Autodesk Inventor part; units mm, degrees
ref_plane "YZ Plane" through (0, 0, 0) normal (1, 0, 0) x (0, 1, 0)
ref_plane "XZ Plane" through (0, 0, 0) normal (0, 1, 0) x (-1, 0, 0)
ref_plane "XY Plane" through (0, 0, 0) normal (0, 0, 1) x (1, 0, 0)
sketch "Sketch1" plane through (0, 0, 0) normal (1, 0, 0) x (0, 1, 0)
  line L0 (0, 0) -> (39.8649, 0)
  line L1 (39.8649, 0) -> (39.8649, -16.6447)
  line L2 (39.8649, -16.6447) -> (37.3249, -16.6447)
  line L3 (37.3249, -16.6447) -> (37.3249, -5.715)
  line L4 (34.1499, -2.54) -> (0, -2.54)
  line L5 (0, -2.54) -> (0, 0)
  arc A0 (37.3249, -5.715) -> (34.1499, -2.54) centre (34.1499, -5.715) ccw
  dimension "d0" = 2.54
  dimension "d1" = 3.175
extrude "Extrusion1" add sketch "Sketch1" along normal blind 2.54
properties part number "allen key"
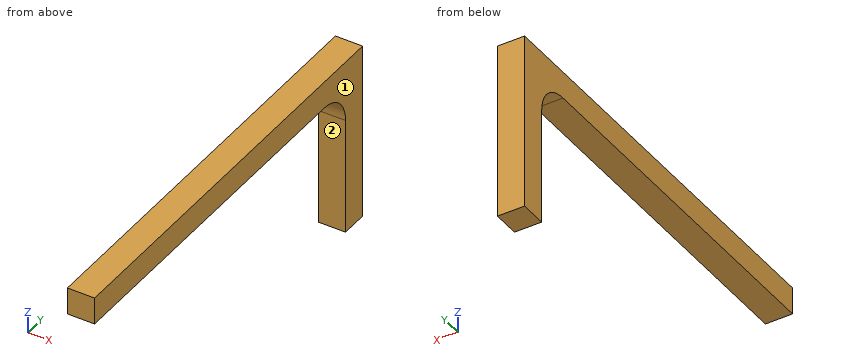
For this review, take the finished solid that the model builds, in its own axes (mm). Face numbers are marked on the shaded views. A direction names the side the tool comes from. Coordinates: 2 decimals unless noted, no trailing zeros. Order: outer loops, then holes, each group sorted by start corner. A loop starts at its lowest first (then second) coordinate and runs counter-clockwise, first axis right, second up. Notation, with made-up numbers: (40, 19.5) - (45, 19.5) arc R18 ccw to (45, 36.5) - close; hole circle Ø2 at (73, -30). An arc over 180 degrees is marked (long way). Answer as CSV lines item,"result". Start each with the question number.
1) Add section B-B (z = -12.5). State the section outline as (x, y) points, then the cut area to 3 significant figures.
2) Insertion check: P1, Ø5, axis at y = 34, z = -8.5, coming from the +X side. The pin has a flat end and moves straight along its axis. Give the tip position at first contact, or say it passes through.
3) Add section C-C (y = 28.5). State the section outline as (x, z) points.
4) Machinability: for the marked faces 1 and 2, which of the approach directions +Z, -Z, +X, -X, +Y, -Y give a long, thin tool a straight path to every point of the face, cutting with its end or side? Answer none if there is none.
5) Add section A-A (x = 2.1). State the section outline as (y, z) points (3 decimals), then the cut area to 3 significant figures.
6) To check wall thickness, follow line 1 along Z through (x, y) = (0.5, 3); line 2 along Y through (x, z) = (0.6, -12.25); line 3 along Z through (x, y) = (1.75, 35). State the ranges of each line that lie inside material, in increasing order. Write a range as [from, to].
Result:
1,outline,"(0, 37.32) - (2.54, 37.32) - (2.54, 39.86) - (0, 39.86) - close"
1,area,"6.45 mm^2"
2,P1,"through"
3,outline,"(0, -2.54) - (2.54, -2.54) - (2.54, 0) - (0, 0) - close"
4,face 1,"+Z, -Z, +X, +Y, -Y"
4,face 2,"-Z, +X, -X, -Y"
5,outline,"(0, -2.54) - (34.15, -2.54) arc R3.175 cw to (37.325, -5.715) - (37.325, -16.645) - (39.865, -16.645) - (39.865, 0) - (0, 0) - close"
5,area,"139 mm^2"
6,line 1,"[-2.54, 0]"
6,line 2,"[37.32, 39.86]"
6,line 3,"[-2.66, 0]"
